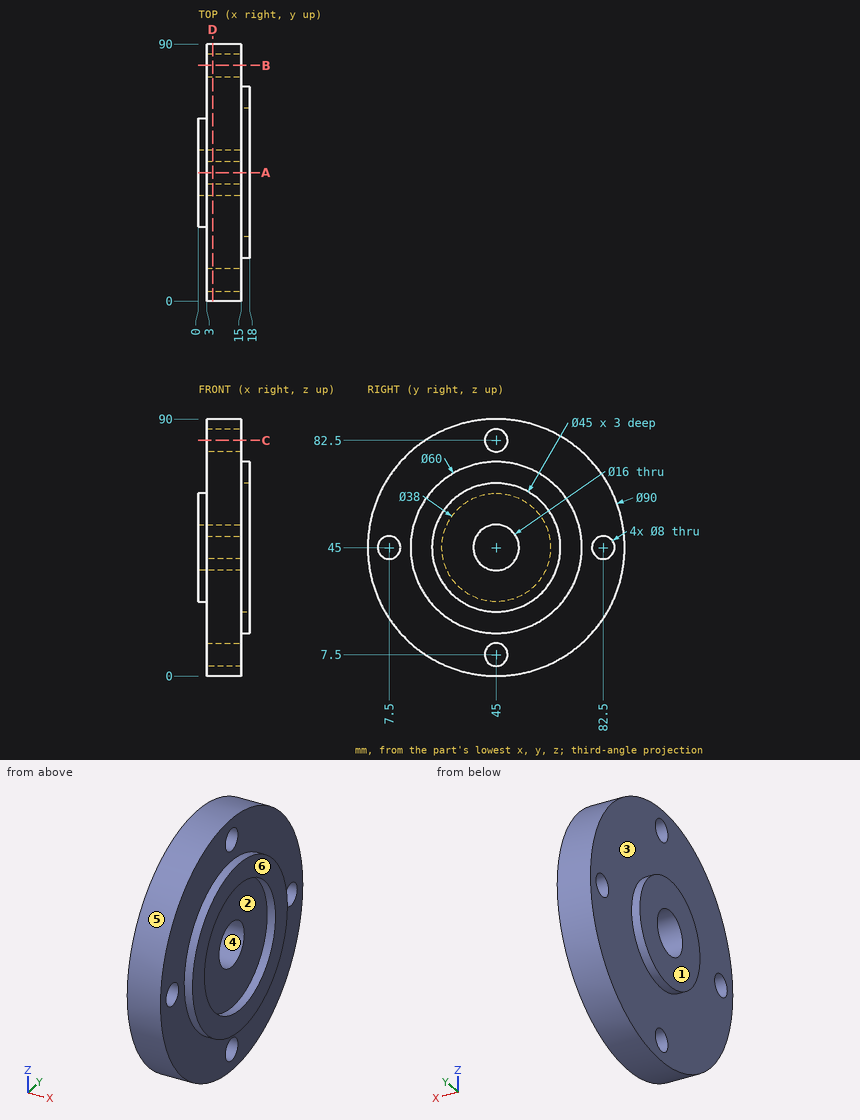
Source: three-view drawing plus pictorial views. Frame: mm from the lowest corner of the part. A direction names the side the tool comes from. Coordinates: 2 decimals unless noted, no trailing zeros. Write each loop counter-clockwise with the first axis right and the second up, starting at its lowest first coordinate (ties: lowest second). Pieces come first, ordered by that corner, then holes. Notation, with made-up numbers: (71, 66) -> (110, 66) arc R16 ccw to (110, 86) -> close; hole circle Ø1 at (19.25, 51.25). An arc over 180 degrees is marked (long way). Write each question's results on one line, items separated by ' | '.
Item 1: Pin query (flat end, axial travel): pin 1 Ø2 at (x, y) = (10, 63.5) entering from +Z; pin 2 Ø13.5 at (y, z) = (49.5, 51) entering from +X; pin 3 Ø6.5 at (y, z) = (45, 7.5) entering from -X; pin 4 Ø10 at (x, y) = (7.5, 39.5) entering from +Z. Return the tip coordinate at first contact, or that it passes through.
Conclusion:
pin 1: stops at z = 86.46 | pin 2: stops at x = 15 | pin 3: passes through | pin 4: stops at z = 90
Item 2: Section query B-B on y = 82.5. Return loops of the section in (x, z), plus the area to 3 significant figures.
Conclusion:
outline: (3, 20.13) -> (15, 20.13) -> (15, 41) -> (3, 41) -> close; (3, 49) -> (15, 49) -> (15, 69.87) -> (3, 69.87) -> close | area: 501 mm^2
Item 3: Section query D-D on x = 5. Return loops of the section in (y, z).
Conclusion:
outline: circle Ø90 at (45, 45); hole circle Ø8 at (7.5, 45); hole circle Ø16 at (45, 45); hole circle Ø8 at (45, 7.5); hole circle Ø8 at (45, 82.5); hole circle Ø8 at (82.5, 45)
Item 4: Section query A-A on y = 45. Return loops of the section in (x, z), plus the area to 3 significant figures.
Conclusion:
outline: (0, 26) -> (3, 26) -> (3, 11.5) -> (15, 11.5) -> (15, 15) -> (18, 15) -> (18, 22.5) -> (15, 22.5) -> (15, 37) -> (0, 37) -> close; (0, 53) -> (15, 53) -> (15, 67.5) -> (18, 67.5) -> (18, 75) -> (15, 75) -> (15, 78.5) -> (3, 78.5) -> (3, 64) -> (0, 64) -> close; (3, 0) -> (15, 0) -> (15, 3.5) -> (3, 3.5) -> close; (3, 86.5) -> (15, 86.5) -> (15, 90) -> (3, 90) -> close | area: 807 mm^2
Item 5: Mould query, pull axis Y, two halves, no side actions, for the marked faces 4, 5 and 6. Classes: +Y half, -Y half, draft (parallel to the pull), parting line (faces both ways), or undercut.
Conclusion:
face 4: undercut | face 5: parting line | face 6: draft
Item 6: Set-up query: the marked faces 1, 2 and 3. Return all of +Z, -Z, +X, -X, +Y, -Y with unobstructed straight access to the full face (end or side cutting, diameter ignored); none if empty.
Conclusion:
face 1: +Z, -Z, -X, +Y, -Y | face 2: +X | face 3: -X
Item 7: Material intervals for probe 1 along Y at (x, z) = (17.15, 45); probe 2 along X at (y, z) = (30.5, 74); probe 3 along Z at (x, y) = (12.5, 80.5), sorted ascending.
Conclusion:
probe 1: y = 15 to 22.5, 67.5 to 75 | probe 2: x = 3 to 15 | probe 3: z = 17.35 to 41.54, 48.46 to 72.65
